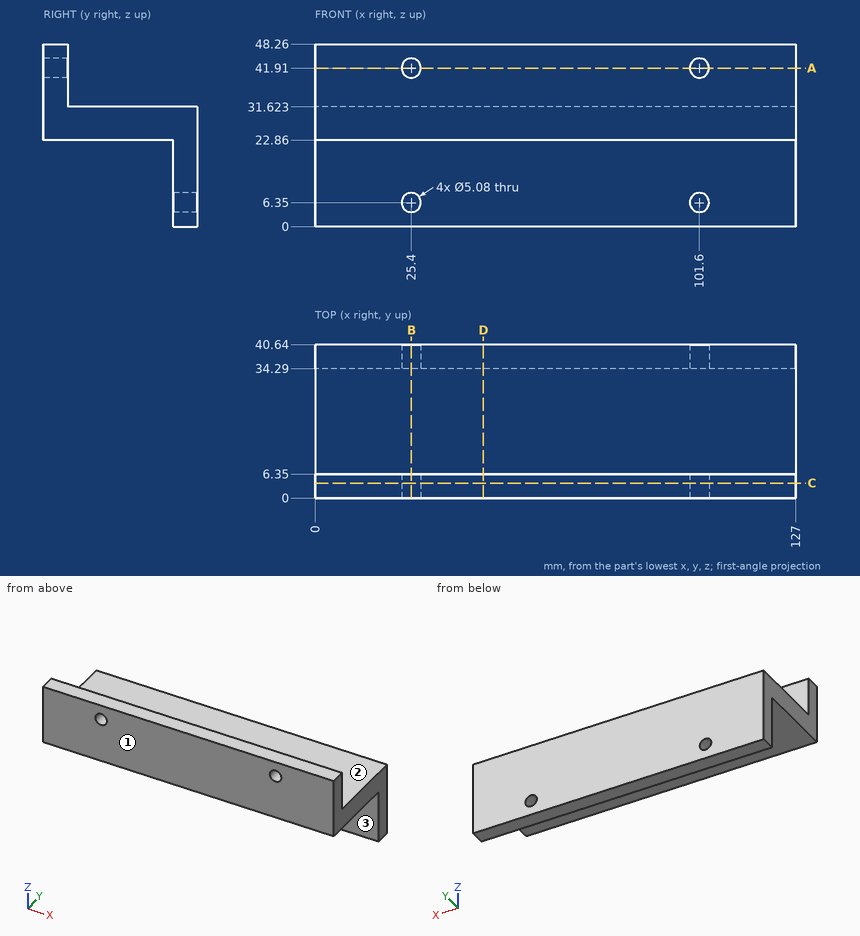
The drawing under review shows one solid part. Ordinate dimensions are in mm from its lowest x, y, z. A direction names the side the tool comes from. Round coordinates to 2 decimals unless told otherwise and drop trailing zeros. Write each loop counter-clockwise with the first axis right and the second up, starting at its lowest first coordinate (ties: lowest second). Pieces come first, ordered by that corner, then holes. Notation, with made-up numbers: (41, 13.25) - (94, 13.25) arc R21 ccw to (94, 20.25) - close; hole circle Ø5 at (85.25, 18). An arc over 180 degrees is marked (long way). Use a Markdown table: item, result. Add a question column.
1. For the marked faces 1, 2 and 3, list the 3-axis set-ups (+Z, -Z, +X, -X, +Y, -Y) from which the entire face can be reached by the end or side of a thin tool; tool diameter is ignored.
2. We need section A-A (z = 41.91). State the section outline as (x, y) points.
3. We need section C-C (y = 4). State the section outline as (x, z) points, then the cut area to 3 significant figures.
4. Clearance check with flat-ended pins moving along their axes: pin 1 (25 mm diameter, centred on x = 50.5, z = 9.5, fed in from -Y); pin 2 (6 mm diameter, centred on x = 86.5, z = 38, fed in from +Y); pin 3 (3 mm diameter, centred on x = 70, y = 18, fed in from -Z). State where each tip first meets the part, or that it passes through.
5. Wall thickness on probe 1 along X at (y, z) = (39, 6); probe 2 along X at (y, z) = (3, 41); probe 3 along Z at (x, y) = (101.6, 37.75): over which ranges is each line inside the solid? List them lowest first.
6. We need section D-D (x = 44.5). State the section outline as (y, z) points.
7. We need section B-B (x = 25.4). State the section outline as (y, z) points.
Output:
| question | item | result |
|---|---|---|
| 1 | face 1 | +Z, -Z, +X, -X, -Y |
| 1 | face 2 | +Z, +X, -X, +Y |
| 1 | face 3 | -Z, +X, -X, -Y |
| 2 | outline | (0, 0) - (22.86, 0) - (22.86, 6.35) - (0, 6.35) - close; (27.94, 0) - (99.06, 0) - (99.06, 6.35) - (27.94, 6.35) - close; (104.14, 0) - (127, 0) - (127, 6.35) - (104.14, 6.35) - close |
| 3 | outline | (0, 22.86) - (127, 22.86) - (127, 48.26) - (0, 48.26) - close; hole circle Ø5.08 at (25.4, 41.91); hole circle Ø5.08 at (101.6, 41.91) |
| 3 | area | 3,190 mm2 |
| 4 | pin 1 | stops at y = 34.29 |
| 4 | pin 2 | stops at y = 6.35 |
| 4 | pin 3 | stops at z = 22.86 |
| 5 | probe 1 | x = 0 to 22.88, 27.92 to 99.08, 104.12 to 127 |
| 5 | probe 2 | x = 0 to 23.03, 27.77 to 99.23, 103.97 to 127 |
| 5 | probe 3 | z = 0 to 3.81, 8.89 to 31.62 |
| 6 | outline | (0, 22.86) - (34.29, 22.86) - (34.29, 0) - (40.64, 0) - (40.64, 31.62) - (6.35, 31.62) - (6.35, 48.26) - (0, 48.26) - close |
| 7 | outline | (0, 22.86) - (34.29, 22.86) - (34.29, 8.89) - (40.64, 8.89) - (40.64, 31.62) - (6.35, 31.62) - (6.35, 39.37) - (0, 39.37) - close; (0, 44.45) - (6.35, 44.45) - (6.35, 48.26) - (0, 48.26) - close; (34.29, 0) - (40.64, 0) - (40.64, 3.81) - (34.29, 3.81) - close |
